Check sheet for the modelled part. Datum: model origin and axes. Units: mm. A direction names the side the tool comes from. Coordinates: 2 decimals unless noted, no trailing zeros. Order: outer loops, then holes, each group sorted by start corner. A loop starts at its lowest first (then second) coordinate and runs counter-clockwise, first axis right, second up. Notation, with made-up numbers: (67, -35.5) -> (84, -35.5) arc R36 ccw to (84, -0.5) -> close; hole circle Ø2 at (60.5, 89.25). An arc over 180 degrees is marked (long way). Put each result on its own line as item: value. Start each with the question number.
```python
from build123d import *

# Parameters (mm, degrees)
F0_W     = 103.98125
F0_H     = 50.00625
F0_W_2   = 97.63125
F0_H_2   = 43.65625
F0_W_3   = 38.1
F0_H_3   = 40.48125
F1_DEPTH = 4.7625
F2_DEPTH = 14.2875
F3_DEPTH = 17.4625
F4_R     = 2.794
F4_R_2   = 2.032
F5_DEPTH = 3.175
F6_DEPTH = 14.2875


with BuildPart() as f1:
    # F0 (on Top) → F1 (new body)
    with BuildSketch(Plane.XY):
        with Locations((51.990625, 25.003125)):
            Rectangle(F0_W, F0_H)
        with Locations((51.990625, 25.003125)):
            Rectangle(F0_W_2, F0_H_2, mode=Mode.SUBTRACT)
        with Locations((51.990625, 25.003125)):
            Rectangle(F0_W_2, F0_H_2)
        with Locations((28.575, 25.003125)):
            Rectangle(F0_W_3, F0_H_3, mode=Mode.SUBTRACT)
        with Locations((75.40625, 25.003125)):
            Rectangle(F0_W_3, F0_H_3, mode=Mode.SUBTRACT)
        with Locations((28.575, 25.003125)):
            Rectangle(F0_W_3, F0_H_3)
        with Locations((75.40625, 25.003125)):
            Rectangle(F0_W_3, F0_H_3)
    extrude(amount=F1_DEPTH)

    # F0 (on Top) → F2 (join)
    with BuildSketch(Plane.XY):
        with Locations((51.990625, 25.003125)):
            Rectangle(F0_W, F0_H)
        with Locations((51.990625, 25.003125)):
            Rectangle(F0_W_2, F0_H_2, mode=Mode.SUBTRACT)
        with Locations((51.990625, 25.003125)):
            Rectangle(F0_W_2, F0_H_2)
        with Locations((28.575, 25.003125)):
            Rectangle(F0_W_3, F0_H_3, mode=Mode.SUBTRACT)
        with Locations((75.40625, 25.003125)):
            Rectangle(F0_W_3, F0_H_3, mode=Mode.SUBTRACT)
    extrude(amount=F2_DEPTH)

    # F0 (on Top) → F3 (join)
    with BuildSketch(Plane.XY):
        with Locations((51.990625, 25.003125)):
            Rectangle(F0_W, F0_H)
        with Locations((51.990625, 25.003125)):
            Rectangle(F0_W_2, F0_H_2, mode=Mode.SUBTRACT)
    extrude(amount=F3_DEPTH)

    # F4 (on face) → F5 (cut)
    with BuildSketch(Plane.XY.offset(14.2875)):
        with Locations((6.35, 43.799125)):
            Circle(F4_R)
        with Locations((6.35, 43.799125)):
            Circle(F4_R_2, mode=Mode.SUBTRACT)
        with Locations((6.35, 6.207125)):
            Circle(F4_R)
        with Locations((6.35, 6.207125)):
            Circle(F4_R_2, mode=Mode.SUBTRACT)
        with Locations((97.63125, 43.799125)):
            Circle(F4_R)
        with Locations((97.63125, 43.799125)):
            Circle(F4_R_2, mode=Mode.SUBTRACT)
        with Locations((97.63125, 6.207125)):
            Circle(F4_R)
        with Locations((97.63125, 6.207125)):
            Circle(F4_R_2, mode=Mode.SUBTRACT)
    extrude(amount=-F5_DEPTH, mode=Mode.SUBTRACT)

    # F6 (cut, through all): faces of the model
    f6_faces = [f1.faces().sort_by_distance(p)[0] for p in [
        (6.35, 43.799125, 14.2875),
        (97.63125, 43.799125, 14.2875),
        (97.63125, 6.207125, 14.2875),
        (6.35, 6.207125, 14.2875),
    ]]
    extrude(f6_faces, amount=-F6_DEPTH, mode=Mode.SUBTRACT)


solid = f1.part
```
1) Scan lines: line 1 along Y through (x, z) = (6.35, 6); line 2 along Y through (x, z) = (6.35, 13.3); line 3 along X through (y, z) = (26, 7.25) (3 decimals). Record each from-to range of solid material in increasing order. Write a range as [from, to].
2) Access from +Z, -Z, +X, -X, +Y, -Y to the whole of each face (thin tool, end or side, straight path). Record for faces 1 (the flat face through (75, 25, 4.762)), 2 (the cylindrical face through (99.51, 5.43, 5.63)).
3) Sectioned sample at D-D (x = 75). Record the boundary of the cut face in (y, z) (1 decimal).
4) Sectioned sample at A-A (x = 6.35). State how many separate pieces and enclosed holes the cut face has, plus the area to 3 significant figures.
5) Sectioned sample at C-C (y = 13.5). Record the boundary of the cut face in (x, z) (1 decimal), plus the area to 3 significant figures.
6) Mould release check, pull along Y, two halves, no side actions. Record for faces 3 (the flat face through (51, 0, 9)), 4 (the flat face through (51, 50.006, 9)), 5 (the flat face through (7, 4, 11.112)): +Y half, -Y half, draft (parallel to the pull), parting line (faces both ways), or undercut.
7) Gauge pin test, flat ends, axial feed: pin 1 (6.5 mm diameter, centred on x = 6.35, y = 6.21, fed in from +Z); pin 2 (1.7 mm diameter, centred on x = 5.5, y = 43.5, fed in from +Z); pin 3 (19 mm diameter, centred on x = 30.5, y = 16.5, fed in from +Z); pin 4 (4.5 mm diameter, centred on x = 6.35, y = 6.21, fed in from +Z). Record the tip position at first contact, or that the pin passes through.
Entries:
1. line 1: y = [0, 4.18], [8.24, 41.77], [45.83, 50.01]
1. line 2: y = [0, 3.41], [9, 41.01], [46.59, 50.01]
1. line 3: x = [0, 9.525], [47.625, 56.356], [94.456, 103.981]
2. face 1: +Z
2. face 2: +Z, -Z
3. outline: (0, 0) -> (50, 0) -> (50, 17.5) -> (46.8, 17.5) -> (46.8, 14.3) -> (45.2, 14.3) -> (45.2, 4.8) -> (4.8, 4.8) -> (4.8, 14.3) -> (3.2, 14.3) -> (3.2, 17.5) -> (0, 17.5) -> close
4. separate pieces: 3
4. enclosed holes: 0
4. area: 609 mm2
5. outline: (0, 0) -> (104, 0) -> (104, 17.5) -> (100.8, 17.5) -> (100.8, 14.3) -> (94.5, 14.3) -> (94.5, 4.8) -> (56.4, 4.8) -> (56.4, 14.3) -> (47.6, 14.3) -> (47.6, 4.8) -> (9.5, 4.8) -> (9.5, 14.3) -> (3.2, 14.3) -> (3.2, 17.5) -> (0, 17.5) -> close
5. area: 780 mm2
6. face 3: -Y half
6. face 4: +Y half
6. face 5: undercut
7. pin 1: stops at z = 17.46
7. pin 2: passes through
7. pin 3: stops at z = 4.76
7. pin 4: stops at z = 11.11
